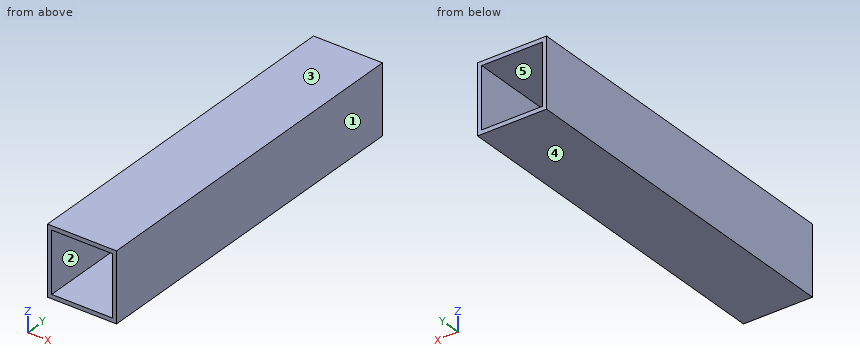
from build123d import *

# Parameters (mm, degrees)
BOSS_EXTRUDE1_DEPTH      = 65
BOSS_EXTRUDE1_DEPTH_BACK = 65
SKETCH1_W                = 25
SKETCH1_H                = 25
SKETCH1_W_2              = 22
SKETCH1_H_2              = 22


with BuildPart() as part:
    # Sketch1 → Boss-Extrude1 (new, two sides: drawn at the far end of the back side and taken through both)
    with BuildSketch(Plane(origin=(0, 0, 0), x_dir=(1, 0, 0), z_dir=(0, 1, 0)).offset(-BOSS_EXTRUDE1_DEPTH_BACK)):
        Rectangle(SKETCH1_W, SKETCH1_H)
        Rectangle(SKETCH1_W_2, SKETCH1_H_2, mode=Mode.SUBTRACT)
    extrude(amount=BOSS_EXTRUDE1_DEPTH + BOSS_EXTRUDE1_DEPTH_BACK)


solid = part.part
CAD build for the part. Positions are in the model's coordinates, mm. Face numbers are marked on the shaded views. A direction names the side the tool comes from. Give positions to 0.01 mm unless a question says otherwise; leave off trailing zeros. Loops run counter-clockwise (first coordinate to the right, second up) from the corner with the lowest first, then second, coordinate; pieces in that order, holes last. Notation, with made-up numbers: M 67.5,-26 L 97.5,-26 A21 ccw 97.5,-8 Z; hole C 41.5,56.25 d6. An arc over 180 degrees is marked long. Answer in a Markdown table with one row per item. Add a question column.
Item 1: Band-saw the part on C-C on y = -18. Give the cut face in (x, z), then the cut area to 3 significant figures.
Item 2: Probe probe 1 along Z at (x, y) = (-8.5, -16.5). List the from-to ranges inside material, lowest first.
Item 3: Mould opens along X. For the marked faces 1, 2 and 3 say: +X half, -X half, draft (parallel to the pull), parting line (faces both ways), or undercut.
Item 4: Band-saw the part on B-B on x = 4. Give the cut face in (y, z).
Item 5: Drop a flat-ended pin along its axis: P1, Ø1, axis at x = 7.5, z = -9.5, coming from the +Y side. Give the stop position or say it passes through.
Item 6: Band-saw the part on A-A on z = -4. Give the cut face in (x, y), then the cut area to 3 significant figures.
Item 7: Tool access for the marked faces 4 and 5: list every direction of +Z, -Z, +X, -X, +Y, -Y with a clear straight run to the whole face (end or side of a thin tool).
Reply:
| question | item | result |
|---|---|---|
| 1 | outline | M -12.5,-12.5 L 12.5,-12.5 L 12.5,12.5 L -12.5,12.5 Z; hole M -11,-11 L 11,-11 L 11,11 L -11,11 Z |
| 1 | area | 141 mm^2 |
| 2 | probe 1 | z = -12.5 to -11, 11 to 12.5 |
| 3 | face 1 | +X half |
| 3 | face 2 | undercut |
| 3 | face 3 | draft |
| 4 | outline | M -65,-12.5 L 65,-12.5 L 65,-11 L -65,-11 Z; M -65,11 L 65,11 L 65,12.5 L -65,12.5 Z |
| 5 | P1 | passes through |
| 6 | outline | M -12.5,-65 L -11,-65 L -11,65 L -12.5,65 Z; M 11,-65 L 12.5,-65 L 12.5,65 L 11,65 Z |
| 6 | area | 390 mm^2 |
| 7 | face 4 | -Z, +X, -X, +Y, -Y |
| 7 | face 5 | +Y, -Y |
